```python
from build123d import *

# Parameters (mm, degrees)
BOSS_EXTRUDE1_DEPTH     = 41
BOSS_EXTRUDE2_REACH     = 50.098
SKETCH2_R               = 1
SKETCH4_W               = 5.5
SKETCH4_H               = 13.1
SKETCH4_R               = 1
CUT_EXTRUDE1_DEPTH      = 7
BOSS_EXTRUDE4_REACH     = 50.098
SKETCH6_W               = 5.5
SKETCH6_H               = 2.85
CUT_EXTRUDE2_DEPTH      = 48.846865116
CUT_EXTRUDE2_DEPTH_BACK = 48.846865116
SKETCH7_W               = 16
SKETCH7_H               = 5.4


with BuildPart() as part:
    # Sketch1 → Boss-Extrude1 (new body)
    with BuildSketch(Plane(origin=(0, 0, 0), x_dir=(0, 0, -1), z_dir=(1, 0, 0))):
        with BuildLine():
            Line((-8.55, 0), (-6.55, 0))
            ThreePointArc((-6.55, 0), (0, -6.55), (6.55, 0))
            Line((6.55, 0), (8.55, 0))
            ThreePointArc((8.55, 0), (15.1, -6.55), (21.65, 0))
            Line((21.65, 0), (23.65, 0))
            Line((23.65, 0), (23.65, -8.55))
            Line((23.65, -8.55), (-23.65, -8.55))
            Line((-23.65, -8.55), (-23.65, 0))
            Line((-23.65, 0), (-21.65, 0))
            ThreePointArc((-21.65, 0), (-15.1, -6.55), (-8.55, 0))
        make_face()
    extrude(amount=BOSS_EXTRUDE1_DEPTH)

    # Sketch2 → Boss-Extrude2 (add, up to next)
    with BuildSketch(Plane(origin=(0, 0, 0), x_dir=(1, 0, 0), z_dir=(0, 1, 0)), mode=Mode.PRIVATE) as boss_extrude2_sk1:
        with Locations(Location((6.6, 3.7, 0), (0, 0, 270))):
            Circle(SKETCH2_R)
    boss_extrude2_tool1 = extrude(boss_extrude2_sk1.sketch, amount=-BOSS_EXTRUDE2_REACH, mode=Mode.PRIVATE) - part.part
    # Sketch2 → Boss-Extrude2 (add, up to next)
    with BuildSketch(Plane(origin=(0, 0, 0), x_dir=(1, 0, 0), z_dir=(0, 1, 0)), mode=Mode.PRIVATE) as boss_extrude2_sk2:
        with Locations(Location((6.6, -3.7, 0), (0, 0, 270))):
            Circle(SKETCH2_R)
    boss_extrude2_tool2 = extrude(boss_extrude2_sk2.sketch, amount=-BOSS_EXTRUDE2_REACH, mode=Mode.PRIVATE) - part.part
    # Sketch2 → Boss-Extrude2 (add, up to next)
    with BuildSketch(Plane(origin=(0, 0, 0), x_dir=(1, 0, 0), z_dir=(0, 1, 0)), mode=Mode.PRIVATE) as boss_extrude2_sk3:
        with Locations(Location((6.6, -11.4, 0), (0, 0, 270))):
            Circle(SKETCH2_R)
    boss_extrude2_tool3 = extrude(boss_extrude2_sk3.sketch, amount=-BOSS_EXTRUDE2_REACH, mode=Mode.PRIVATE) - part.part
    # Sketch2 → Boss-Extrude2 (add, up to next)
    with BuildSketch(Plane(origin=(0, 0, 0), x_dir=(1, 0, 0), z_dir=(0, 1, 0)), mode=Mode.PRIVATE) as boss_extrude2_sk4:
        with Locations(Location((6.6, -18.8, 0), (0, 0, 270))):
            Circle(SKETCH2_R)
    boss_extrude2_tool4 = extrude(boss_extrude2_sk4.sketch, amount=-BOSS_EXTRUDE2_REACH, mode=Mode.PRIVATE) - part.part
    # Sketch2 → Boss-Extrude2 (add, up to next)
    with BuildSketch(Plane(origin=(0, 0, 0), x_dir=(1, 0, 0), z_dir=(0, 1, 0)), mode=Mode.PRIVATE) as boss_extrude2_sk5:
        with Locations(Location((6.6, 18.8, 0), (0, 0, 270))):
            Circle(SKETCH2_R)
    boss_extrude2_tool5 = extrude(boss_extrude2_sk5.sketch, amount=-BOSS_EXTRUDE2_REACH, mode=Mode.PRIVATE) - part.part
    # Sketch2 → Boss-Extrude2 (add, up to next)
    with BuildSketch(Plane(origin=(0, 0, 0), x_dir=(1, 0, 0), z_dir=(0, 1, 0)), mode=Mode.PRIVATE) as boss_extrude2_sk6:
        with Locations(Location((6.6, 11.4, 0), (0, 0, 270))):
            Circle(SKETCH2_R)
    boss_extrude2_tool6 = extrude(boss_extrude2_sk6.sketch, amount=-BOSS_EXTRUDE2_REACH, mode=Mode.PRIVATE) - part.part
    add(boss_extrude2_tool1.solids().sort_by_distance((6.6, 0, -3.7))[0])
    add(boss_extrude2_tool2.solids().sort_by_distance((6.6, 0, 3.7))[0])
    add(boss_extrude2_tool3.solids().sort_by_distance((6.6, 0, 11.4))[0])
    add(boss_extrude2_tool4.solids().sort_by_distance((6.6, 0, 18.8))[0])
    add(boss_extrude2_tool5.solids().sort_by_distance((6.6, 0, -18.8))[0])
    add(boss_extrude2_tool6.solids().sort_by_distance((6.6, 0, -11.4))[0])

    # Sketch4 → Cut-Extrude1 (cut)
    # profile 1 of 3: a face of its own
    with BuildSketch(Plane(origin=(0, 0, 0), x_dir=(1, 0, 0), z_dir=(0, 1, 0))):
        with Locations((6.6, 0)):
            Rectangle(SKETCH4_W, SKETCH4_H)
        with Locations(Location((6.6, 3.7, 0), (0, 0, 270))):
            Circle(SKETCH4_R, mode=Mode.SUBTRACT)
        with Locations(Location((6.6, -3.7, 0), (0, 0, 270))):
            Circle(SKETCH4_R, mode=Mode.SUBTRACT)
    # profile 2 of 3: a face of its own
    with BuildSketch(Plane(origin=(0, 0, 0), x_dir=(1, 0, 0), z_dir=(0, 1, 0))):
        with Locations((6.6, -15.1)):
            Rectangle(SKETCH4_W, SKETCH4_H)
        with Locations(Location((6.6, -11.4, 0), (0, 0, 90))):
            Circle(SKETCH4_R, mode=Mode.SUBTRACT)
        with Locations(Location((6.6, -18.8, 0), (0, 0, 90))):
            Circle(SKETCH4_R, mode=Mode.SUBTRACT)
    # profile 3 of 3: a face of its own
    with BuildSketch(Plane(origin=(0, 0, 0), x_dir=(1, 0, 0), z_dir=(0, 1, 0))):
        with Locations((6.6, 15.1)):
            Rectangle(SKETCH4_W, SKETCH4_H)
        with Locations(Location((6.6, 11.4, 0), (0, 0, 90))):
            Circle(SKETCH4_R, mode=Mode.SUBTRACT)
        with Locations(Location((6.6, 18.8, 0), (0, 0, 90))):
            Circle(SKETCH4_R, mode=Mode.SUBTRACT)
    extrude(amount=-CUT_EXTRUDE1_DEPTH, mode=Mode.SUBTRACT)

    # Boss-Extrude4: up to this face of the body (flat: up to its plane)
    boss_extrude4_end = Plane(part.part.faces().sort_by_distance((6.6, -7, -15.1))[0])
    # Sketch6 → Boss-Extrude4 (add, up to the picked face)
    with BuildSketch(Plane(origin=(0, 0, 0), x_dir=(1, 0, 0), z_dir=(0, 1, 0)), mode=Mode.PRIVATE) as boss_extrude4_sk1:
        with Locations((6.6, -5.125)):
            Rectangle(SKETCH6_W, SKETCH6_H)
    boss_extrude4_tool1 = split(extrude(boss_extrude4_sk1.sketch, amount=-BOSS_EXTRUDE4_REACH, mode=Mode.PRIVATE), bisect_by=boss_extrude4_end, keep=Keep.BOTH, mode=Mode.PRIVATE)
    # Sketch6 → Boss-Extrude4 (add, up to the picked face)
    with BuildSketch(Plane(origin=(0, 0, 0), x_dir=(1, 0, 0), z_dir=(0, 1, 0)), mode=Mode.PRIVATE) as boss_extrude4_sk2:
        with Locations((6.6, 5.125)):
            Rectangle(SKETCH6_W, SKETCH6_H)
    boss_extrude4_tool2 = split(extrude(boss_extrude4_sk2.sketch, amount=-BOSS_EXTRUDE4_REACH, mode=Mode.PRIVATE), bisect_by=boss_extrude4_end, keep=Keep.BOTH, mode=Mode.PRIVATE)
    # Sketch6 → Boss-Extrude4 (add, up to the picked face)
    with BuildSketch(Plane(origin=(0, 0, 0), x_dir=(1, 0, 0), z_dir=(0, 1, 0)), mode=Mode.PRIVATE) as boss_extrude4_sk3:
        with Locations((6.6, -20.225)):
            Rectangle(SKETCH6_W, SKETCH6_H)
    boss_extrude4_tool3 = split(extrude(boss_extrude4_sk3.sketch, amount=-BOSS_EXTRUDE4_REACH, mode=Mode.PRIVATE), bisect_by=boss_extrude4_end, keep=Keep.BOTH, mode=Mode.PRIVATE)
    # Sketch6 → Boss-Extrude4 (add, up to the picked face)
    with BuildSketch(Plane(origin=(0, 0, 0), x_dir=(1, 0, 0), z_dir=(0, 1, 0)), mode=Mode.PRIVATE) as boss_extrude4_sk4:
        with Locations((6.6, -9.975)):
            Rectangle(SKETCH6_W, SKETCH6_H)
    boss_extrude4_tool4 = split(extrude(boss_extrude4_sk4.sketch, amount=-BOSS_EXTRUDE4_REACH, mode=Mode.PRIVATE), bisect_by=boss_extrude4_end, keep=Keep.BOTH, mode=Mode.PRIVATE)
    # Sketch6 → Boss-Extrude4 (add, up to the picked face)
    with BuildSketch(Plane(origin=(0, 0, 0), x_dir=(1, 0, 0), z_dir=(0, 1, 0)), mode=Mode.PRIVATE) as boss_extrude4_sk5:
        with Locations((6.6, 9.975)):
            Rectangle(SKETCH6_W, SKETCH6_H)
    boss_extrude4_tool5 = split(extrude(boss_extrude4_sk5.sketch, amount=-BOSS_EXTRUDE4_REACH, mode=Mode.PRIVATE), bisect_by=boss_extrude4_end, keep=Keep.BOTH, mode=Mode.PRIVATE)
    # Sketch6 → Boss-Extrude4 (add, up to the picked face)
    with BuildSketch(Plane(origin=(0, 0, 0), x_dir=(1, 0, 0), z_dir=(0, 1, 0)), mode=Mode.PRIVATE) as boss_extrude4_sk6:
        with Locations((6.6, 20.225)):
            Rectangle(SKETCH6_W, SKETCH6_H)
    boss_extrude4_tool6 = split(extrude(boss_extrude4_sk6.sketch, amount=-BOSS_EXTRUDE4_REACH, mode=Mode.PRIVATE), bisect_by=boss_extrude4_end, keep=Keep.BOTH, mode=Mode.PRIVATE)
    add(boss_extrude4_tool1.solids().sort_by(Axis((6.6, 0, 5.125), (0, -1, 0)))[0])
    add(boss_extrude4_tool2.solids().sort_by(Axis((6.6, 0, -5.125), (0, -1, 0)))[0])
    add(boss_extrude4_tool3.solids().sort_by(Axis((6.6, 0, 20.225), (0, -1, 0)))[0])
    add(boss_extrude4_tool4.solids().sort_by(Axis((6.6, 0, 9.975), (0, -1, 0)))[0])
    add(boss_extrude4_tool5.solids().sort_by(Axis((6.6, 0, -9.975), (0, -1, 0)))[0])
    add(boss_extrude4_tool6.solids().sort_by(Axis((6.6, 0, -20.225), (0, -1, 0)))[0])

    # Sketch7 → Cut-Extrude2 (cut, two sides: drawn at the far end of the back side and taken through both)
    with BuildSketch(Plane(origin=(0, -7, 0), x_dir=(1, 0, 0), z_dir=(0, 1, 0)).offset(-CUT_EXTRUDE2_DEPTH_BACK)):
        with Locations((8, 0)):
            Rectangle(SKETCH7_W, SKETCH7_H)
        with Locations((8, -15.1)):
            Rectangle(SKETCH7_W, SKETCH7_H)
        with Locations((8, 15.1)):
            Rectangle(SKETCH7_W, SKETCH7_H)
    extrude(amount=CUT_EXTRUDE2_DEPTH + CUT_EXTRUDE2_DEPTH_BACK, mode=Mode.SUBTRACT)


solid = part.part
```
Source: CAD feature listing. Evaluate the final solid. Frame: model axes, mm. A direction names the side the tool comes from. Give positions to 0.01 mm unless a question says otherwise; leave off trailing zeros. Write each loop counter-clockwise with the first axis right and the second up, starting at its lowest first coordinate (ties: lowest second). Pieces come first, ordered by that corner, then holes. Notation, with made-up numbers: (85, -31.5) - (100, -31.5) arc R23 cw to (100, -18.5) - close; hole circle Ø7 at (-8.75, 46.5). An arc over 180 degrees is marked (long way). One line per item, written item: value. Start each with the question number.
Q1. First-contact query: pin 1 Ø3 at (y, z) = (-4, -10.5) entering from -X; pin 2 Ø3 at (x, z) = (16.5, -15) entering from +Y; pin 3 Ø0.9 at (y, z) = (-1.5, 20.5) entering from +X; pin 4 Ø0.8 at (x, z) = (8, -12) entering from +Y. Flat tips, straight axial feed; report the tip coordinate or a pass-through.
Q2. Material intervals for probe 1 along Z at (x, y) = (9, -1.25); probe 2 along X at (y, z) = (-6.5, 11.5); probe 3 along Z at (x, y) = (15, -6.75), sorted ascending. Write a range as from..to.
Q3. Section query A-A, the plane x = 14. Return the cut outline in (y, z).
Q4. Section query C-C, the plane y = -4.75. Count the separate pieces of the cut face and the enclosed holes in it, then the cut area to 3 significant figures.
Q5. Set-up query: faces 1 (the face through (7.9, -7.3, -17.8)), 2 (the face through (6.6, -3.5, -12.4)), 3 (the face through (9.35, -2, 10)), 4 (the face through (3.85, -2, 10)). Return all of +Z, -Z, +X, -X, +Y, -Y with unobstructed straight access to the full face (end or side cutting, diameter ignored); none if empty.
Q6. Section query D-D, the plane z = 6. Return the cut outline in (x, y), then the cut area to 3 significant figures.
Q7. Draft query along Z for faces 5 (the face through (16, 0, 7)), 6 (the face through (1.9, -3.51, 5.53)), 7 (the face through (20, -4, 23.65)), 8 (the face through (7.9, -7.3, 17.8)). Return one class per face: +Z half, -Z half, draft (parallel to the pull), parting line (faces both ways), or undercut.
Q8. Section query B-B, the plane z = -10.5. Return the cut outline in (x, y), then the cut area to 3 significant figures.
Answer:
1. pin 1: stops at x = 0
1. pin 2: stops at y = -6.35
1. pin 3: stops at x = 9.35
1. pin 4: stops at y = -7
2. probe 1: z = -23.65..-18.8, -11.4..-3.7, 3.7..11.4, 18.8..23.65
2. probe 2: x = 0..3.85, 5.61..7.59, 9.35..41
2. probe 3: z = -23.65..-17.8, -12.4..-2.7, 2.7..12.4, 17.8..23.65
3. outline: (-8.55, -23.65) - (0, -23.65) - (0, -21.65) arc R6.55 cw to (-5.97, -17.8) - (-8.55, -17.8) - close; (-8.55, -12.4) - (-5.97, -12.4) arc R6.55 cw to (0, -8.55) - (0, -6.55) arc R6.55 cw to (-5.97, -2.7) - (-8.55, -2.7) - close; (-8.55, 2.7) - (-5.97, 2.7) arc R6.55 cw to (0, 6.55) - (0, 8.55) arc R6.55 cw to (-5.97, 12.4) - (-8.55, 12.4) - close; (-8.55, 17.8) - (-5.97, 17.8) arc R6.55 cw to (0, 21.65) - (0, 23.65) - (-8.55, 23.65) - close
4. separate pieces: 4
4. enclosed holes: 0
4. area: 866 mm2
5. face 1: -X, +Y, -Y
5. face 2: +Y
5. face 3: +X, +Y
5. face 4: -X, +Y
6. outline: (0, -8.55) - (41, -8.55) - (41, -2.63) - (9.35, -2.63) - (9.35, 0) - (3.85, 0) - (3.85, -2.63) - (0, -2.63) - close
6. area: 257 mm2
7. face 5: draft
7. face 6: undercut
7. face 7: +Z half
7. face 8: undercut
8. outline: (0, -8.55) - (41, -8.55) - (41, -4.66) - (9.35, -4.66) - (9.35, 0) - (3.85, 0) - (3.85, -4.66) - (0, -4.66) - close
8. area: 185 mm2
